from build123d import *

# Parameters (mm, degrees)
SKETCH1_W            = 35
SKETCH1_H            = 105
BOSS_EXTRUDE1_DEPTH  = 6
M4_CLEARANCE_HOLE1_D = 4.8
LPATTERN2_COUNT      = 2
LPATTERN2_PITCH      = 10
SKETCH5_W            = 4.8
SKETCH5_H            = 10
SKETCH5_W_2          = 4.730666207
SKETCH5_H_2          = 10.572708501
CUT_EXTRUDE1_DEPTH   = 88.085432636
SKETCH6_W            = 11.2
SKETCH6_H            = 11.2
CUT_EXTRUDE2_DEPTH   = 4
SKETCH7_W            = 7
SKETCH7_H            = 7
CUT_EXTRUDE3_DEPTH   = 87.970527062
SKETCH8_W            = 8
SKETCH8_H            = 16.2
CUT_EXTRUDE4_DEPTH   = 4
FILLET1_R            = 10
CUT_EXTRUDE5_START   = -6
SKETCH9_W            = 37.049954943
SKETCH9_H            = 41
CUT_EXTRUDE5_DEPTH   = 3
FILLET2_R            = 30
FILLET3_R            = 30


with BuildPart() as part:
    # Sketch1 → Boss-Extrude1 (new body)
    with BuildSketch(Plane(origin=(0, 0, 0), x_dir=(1, 0, 0), z_dir=(0, 1, 0))):
        with Locations((0.111940299, -32.574626866)):
            Rectangle(SKETCH1_W, SKETCH1_H)
    extrude(amount=BOSS_EXTRUDE1_DEPTH)

    # M4 Clearance Hole1 (through all)
    with Locations(Plane(origin=(0, 6, 0), x_dir=(1, 0, 0), z_dir=(0, 1, 0))):
        with Locations((-12.388059701, 14.925373134), (12.611940299, 14.925373134), (12.611940299, -10.074626866), (-12.388059701, -10.074626866)):
            m4_clearance_hole1 = Hole(M4_CLEARANCE_HOLE1_D / 2)

    # LPattern2: M4 Clearance Hole1 ×2
    with Locations(*[(0, 0, i * LPATTERN2_PITCH) for i in range(1, LPATTERN2_COUNT)]):
        add(m4_clearance_hole1, mode=Mode.SUBTRACT)

    # Sketch5 → Cut-Extrude1 (cut, through all)
    with BuildSketch(Plane(origin=(0, 6, 0), x_dir=(1, 0, 0), z_dir=(0, 1, 0))):
        with Locations((-12.388059701, 9.925373134)):
            Rectangle(SKETCH5_W, SKETCH5_H)
        with Locations((-12.388059701, -15.074626866)):
            Rectangle(SKETCH5_W, SKETCH5_H)
        with Locations((12.577273403, 9.639018884)):
            Rectangle(SKETCH5_W_2, SKETCH5_H_2)
        with Locations((12.577273403, -15.360981116)):
            Rectangle(SKETCH5_W_2, SKETCH5_H_2)
    extrude(amount=-CUT_EXTRUDE1_DEPTH, mode=Mode.SUBTRACT)

    # Sketch6 → Cut-Extrude2 (cut)
    with BuildSketch(Plane(origin=(0, 6, 0), x_dir=(1, 0, 0), z_dir=(0, 1, 0))):
        with Locations((0.111940299, -75.074626866)):
            Rectangle(SKETCH6_W, SKETCH6_H)
    extrude(amount=-CUT_EXTRUDE2_DEPTH, mode=Mode.SUBTRACT)

    # Sketch7 → Cut-Extrude3 (cut, through all)
    with BuildSketch(Plane(origin=(0, 2, 0), x_dir=(1, 0, 0), z_dir=(0, 1, 0))):
        with Locations((0.111940299, -75.074626866)):
            Rectangle(SKETCH7_W, SKETCH7_H)
    extrude(amount=-CUT_EXTRUDE3_DEPTH, mode=Mode.SUBTRACT)

    # Sketch8 → Cut-Extrude4 (cut)
    with BuildSketch(Plane(origin=(0, 6, 0), x_dir=(1, 0, 0), z_dir=(0, 1, 0))):
        with Locations((0.111940299, -75.074626866)):
            Rectangle(SKETCH8_W, SKETCH8_H)
    extrude(amount=-CUT_EXTRUDE4_DEPTH, mode=Mode.SUBTRACT)

    # Fillet1
    fillet1_edges = [part.edges().sort_by_distance(p)[0] for p in [
        (17.611940299, 3, 85.074626866),
        (-17.388059701, 3, 85.074626866),
    ]]
    fillet(fillet1_edges, radius=FILLET1_R)

    # Sketch9 → Cut-Extrude5 (cut)
    with BuildSketch(Plane.XZ.offset(CUT_EXTRUDE5_START)):
        with Locations((1.136917771, 64.574626866)):
            Rectangle(SKETCH9_W, SKETCH9_H)
    extrude(amount=CUT_EXTRUDE5_DEPTH, mode=Mode.SUBTRACT)

    # Fillet2
    # the kernel refuses this fillet: 30 mm, written as the material it adds along each edge
    with BuildSketch(Plane(origin=(-17.388059701, 3, 44.074626866), x_dir=(0, 1, 0), z_dir=(1, 0, 0))) as fillet2_piece_1:
        with BuildLine():
            CenterArc((30, 13.076696831), FILLET2_R, 180, 25.841932763)
            Line((0, 13.076696831), (-0.6, 13.076696831))
            Line((-0.6, 13.076696831), (-0.6, 0))
            Line((-0.6, 0), (0, -0.6))
            ThreePointArc((0, -0.6), (1.5, -0.6), (2.46, -0.261533937))
            Line((2.46, -0.261533937), (3, 0))
        make_face()
    extrude(amount=35)

    # Fillet3
    fillet3_edges = [part.edges().sort_by_distance(p)[0] for p in [
        (0.111940299, 6, 44.074626866),
    ]]
    fillet(fillet3_edges, radius=FILLET3_R)


solid = part.part
Design review of the part built by this model. Coordinates are the model's own, in mm. A direction names the side the tool comes from. Coordinates: 2 decimals unless noted, no trailing zeros. Loops run counter-clockwise (first coordinate to the right, second up) from the corner with the lowest first, then second, coordinate; pieces in that order, holes last.
Item 1: Add section C-C (z = 46). Write out the cut boundary in (x, y).
Completed:
outline: (-17.39, 0) - (17.61, 0) - (17.61, 5.03) - (-17.39, 5.03) - close
Item 2: Add section A-A (z = 68.5). Write out the cut boundary in (x, y).
Completed:
outline: (-17.39, 0) - (17.61, 0) - (17.61, 3) - (4.11, 3) - (4.11, 2) - (-3.89, 2) - (-3.89, 3) - (-17.39, 3) - close
Item 3: For faces 5 (the flat face through (0, 3, -19.925)), 6 (the flat face through (-9.988, 3, -10)), list the 3-axis set-ups (+Z, -Z, +X, -X, +Y, -Y) from which the entire face can be reached by the end or side of a thin tool; tool diameter is ignored.
Completed:
face 5: -Z, +X, -X, +Y, -Y
face 6: +Y, -Y
Item 4: Add section B-B (x = -9). Write out the cut boundary in (y, z), and give its area (3 significant figures).
Completed:
outline: (0, -19.93) - (6, -19.93) - (6, 38.42) arc R30 ccw to (4.5, 47.78) arc R30 cw to (3, 57.15) - (3, 84.94) - (0, 84.94) - close
area: 518 mm2
Item 5: Draft analysis for pull direction X (two halves, no side actions). For faces 1 (the cylindrical face through (13.2, 3, -2.6)), 2 (the flat face through (0, 3, 65)), 3 (the cylindrical face through (14.605, 1.521, 82.223)), 4 (the flat face through (0, 2, 71)), state which applies: pulls with the +X half, pulls with the -X half, needs draft (parallel to the pull), parting line crosses it, or undercut.
Completed:
face 1: undercut
face 2: needs draft
face 3: pulls with the +X half
face 4: undercut
Item 6: Wall thickness on L1, parallel to X at y = 0.35, z = 18; L2, parallel to X at y = 2.5, z = 75.5; L3, parallel to Y at x = -13, z = 74.5: over which ranges is each line inside the solid? List them lowest first.
Completed:
L1: x = -17.39 to -14.79, -9.99 to 10.21, 14.94 to 17.61
L2: x = -17.38 to -5.49, 5.71 to 17.6
L3: y = 0 to 3
